Input: part model. Units: mm. Frame: model coordinates. A direction names the side the tool comes from. Coordinates: 2 decimals unless noted, no trailing zeros. Write each loop counter-clockwise with the first axis right and the second up, starting at its lowest first coordinate (ties: lowest second). Pieces come first, ordered by that corner, then holes. Notation, with made-up numbers: (-6, 44) - (4, 44) arc R23 ccw to (4, 64) - close; hole circle Ø7 at (-9.5, -8.75). An arc over 180 degrees is marked (long way). One line per question, with ' | ' between items. Start each with the question number.
1) Section query D-D on z = 8.5. Return loops of the section in (x, y), and give its area (3 significant figures).
2) Draft query along Y for faces 1 (the cylindrical face through (20.472, 0.21, 1.449)), 2 (the flat face through (0, -4.964, 2)), 3 (the flat face through (0, -11, 58)), 4 (the cylindrical face through (-0.16, -13.83, 3.25)). Return one class per face: released by +Y, released by -Y, zero draft, split by the parting line, or undercut.
3) Section query C-C on y = -9.5. Return loops of the section in (x, z).
4) Reachability of faces 5 (the cylindrical face through (20.472, 0.21, 112.551)), 6 (the flat face through (-11.227, -10, 3)), 7 (the flat face through (0, 2, 110)) from +Z, -Z, +X, -X, +Y, -Y: full face, straight path, thin tool, end or side. Return the list, or none.
5) Section query A-A on x = 10. Return loops of the section in (y, z).
6) Line query: line 1 (X direction, y = 2, z = 75.5); line 2 (Z direction, x = -10, y = 7); line 3 (Y direction, x = -17.5, z = 88.5). Output: solid intervals per line, ascending.
7) First-contact query: P1, Ø2.5, axis at y = -12, z = 3.5, coming from the +X side; P2, Ø3, axis at x = -3, z = 54, coming from the +Y side. Flat tips, straight axial feed; report the tip coordinate or a pass-through.
8) Section query B-B on y = 2.75. Return loops of the section in (x, z).
```python
from build123d import *

# Parameters (mm, degrees)
F0_W        = 44
F0_H        = 30
F1_DEPTH    = 114
F2_W        = 35
F2_H        = 105
F3_DEPTH    = 26
F4_R        = 5.08
F5_R        = 2.4528409794
F6_W        = 22.4547982216
F6_H        = 9.9273854867
F7_DEPTH    = 5.08
F8_T1_DEPTH = 22.4547982216


# Not quite as in the source:
# - a fillet or chamfer that OpenCascade refuses, or shapes differently, is made with other operations: its cross-section is extruded or revolved along the edge and cut away or added


with BuildPart() as f1:
    # F0 (on Top) → F1 (new body)
    with BuildSketch(Plane.XY):
        Rectangle(F0_W, F0_H)
    extrude(amount=F1_DEPTH)

    # F2 (on face) → F3 (cut)
    with BuildSketch(Plane(origin=(0, 15, 0), x_dir=(-1, 0, 0), z_dir=(0, 1, 0))):
        with Locations((0.5, 57.5)):
            Rectangle(F2_W, F2_H)
    extrude(amount=-F3_DEPTH, mode=Mode.SUBTRACT)

    # F4
    f4_edges = [f1.edges().sort_by_distance(p)[0] for p in [
        (22, 0, 0),
        (-22, 0, 0),
        (-22, 0, 114),
        (22, 0, 114),
    ]]
    fillet(f4_edges, radius=F4_R)

    # F5
    f5_edges = [f1.edges().sort_by_distance(p)[0] for p in [
        (17, 2, 110),
        (-18, 2, 110),
        (17, 2, 5),
        (-18, 2, 5),
    ]]
    fillet(f5_edges, radius=F5_R)

    # F6 (on face) → F7 (cut)
    with BuildSketch(Plane(origin=(0, 0, 0), x_dir=(1, 0, 0), z_dir=(0, 0, -1))):
        with Locations((0, 9.9273854867)):
            Rectangle(F6_W, F6_H)
    extrude(amount=-F7_DEPTH, mode=Mode.SUBTRACT)

    # F8: fillet of radius 5.08 on 1 edges, made by hand

    # F8_s2 → F8_t1 (join)
    with BuildSketch(Plane.YZ.offset(-11.2273991108)):
        with BuildLine():
            ThreePointArc((-14.89107823, 0.1410866555), (-13.8014493024, 3.2848644314), (-11, 5.08))
            Line((-11, 5.08), (-14.89107823, 5.08))
            Line((-14.89107823, 5.08), (-14.89107823, 0.1410866555))
        make_face()
    extrude(amount=F8_T1_DEPTH)


solid = f1.part
```
Answer key:
1) outline: (-22, -15) - (22, -15) - (22, 15) - (17, 15) - (17, -11) - (-18, -11) - (-18, 15) - (-22, 15) - close | area: 410 mm²
2) face 1: zero draft | face 2: undercut | face 3: released by +Y | face 4: undercut
3) outline: (-22, 5.08) arc R5.08 ccw to (-16.92, 0) - (-11.23, 0) - (-11.23, 5) - (-15.55, 5) arc R2.45 cw to (-18, 7.45) - (-18, 107.55) arc R2.45 cw to (-15.55, 110) - (14.55, 110) arc R2.45 cw to (17, 107.55) - (17, 7.45) arc R2.45 cw to (14.55, 5) - (11.23, 5) - (11.23, 0) - (16.92, 0) arc R5.08 ccw to (22, 5.08) - (22, 108.92) arc R5.08 ccw to (16.92, 114) - (-16.92, 114) arc R5.08 ccw to (-22, 108.92) - close
4) face 5: +Z, +X, +Y, -Y | face 6: -Z | face 7: +Y
5) outline: (-15, 0) - (-14.89, 0) - (-14.89, 0.14) arc R5.08 cw to (-11, 5.08) - (-11, 110) - (15, 110) - (15, 114) - (-15, 114) - close; (-4.96, 0) - (15, 0) - (15, 5) - (-4.96, 5) - close
6) line 1: -22 to -18, 17 to 22 | line 2: 0 to 5, 110 to 114 | line 3: -15 to -11
7) P1: x = 21.99 | P2: y = -11
8) outline: (-22, 5.08) arc R5.08 ccw to (-16.92, 0) - (16.92, 0) arc R5.08 ccw to (22, 5.08) - (22, 108.92) arc R5.08 ccw to (16.92, 114) - (-16.92, 114) arc R5.08 ccw to (-22, 108.92) - close; hole (-18, 7.45) arc R2.45 ccw to (-15.55, 5) - (14.55, 5) arc R2.45 ccw to (17, 7.45) - (17, 107.55) arc R2.45 ccw to (14.55, 110) - (-15.55, 110) arc R2.45 ccw to (-18, 107.55) - close
